```python
from build123d import *

# Parameters (mm, degrees)
SKETCH_2_R           = 2.5
EXTRUDE_4_DEPTH      = 10
SKETCH_3_W           = 45
SKETCH_3_H           = 10
EXTRUDE_5_DEPTH      = 53.5
CUT_EXTRUDE_2_DEPTH  = 62
SKETCH_5_W           = 2
SKETCH_5_H           = 40
EXTRUDE_6_DEPTH      = 4
SKETCH_6_W           = 6
SKETCH_6_H           = 18.13920413
SKETCH_6_H_2         = 19.86079587
EXTRUDE_7_DEPTH      = 2
SKETCH_8_R           = 2
CUT_EXTRUDE_3_DEPTH  = 15
SKETCH_9_W           = 4
SKETCH_9_H           = 2
CUT_EXTRUDE_4_DEPTH  = 8
CUT_EXTRUDE_6_DEPTH  = 70.189906512
CUT_EXTRUDE_7_DEPTH  = 70.189906512
CUT_EXTRUDE_8_DEPTH  = 4
CHAMFER_1_SIZE       = 0.5
CHAMFER_2_SIZE       = 1
FILLET_1_R           = 1
FILLET_2_R           = 1
SKETCH_13_R          = 2.65
CUT_EXTRUDE_9_DEPTH  = 74.226354795
CUT_EXTRUDE_10_DEPTH = 62
SKETCH_15_R          = 2.15
CUT_EXTRUDE_11_DEPTH = 15
SKETCH_16_W          = 9
SKETCH_16_H          = 5
CUT_EXTRUDE_12_DEPTH = 8.5


with BuildPart() as part:
    # Эскиз2 → Бобышка-Вытянуть4 (new body)
    with BuildSketch(Plane.XY):
        with BuildLine():
            Line((-25.592834214, -15.977988248), (-13.092834214, -15.977988248))
            ThreePointArc((-13.092834214, -15.977988248), (-3.092834214, -5.977988248), (6.907165786, -15.977988248))
            Line((6.907165786, -15.977988248), (19.407165786, -15.977988248))
            Line((19.407165786, -15.977988248), (19.407165786, -25.977988248))
            Line((19.407165786, -25.977988248), (-25.592834214, -25.977988248))
            Line((-25.592834214, -25.977988248), (-25.592834214, -15.977988248))
        make_face()
        with Locations((-3.092834214, -15.977988248)):
            Circle(SKETCH_2_R, mode=Mode.SUBTRACT)
    extrude(amount=EXTRUDE_4_DEPTH)

    # Эскиз3 → Бобышка-Вытянуть5 (add)
    with BuildSketch(Plane.XY.offset(10)):
        with Locations((-3.092834214, -20.977988248)):
            Rectangle(SKETCH_3_W, SKETCH_3_H)
    extrude(amount=EXTRUDE_5_DEPTH)

    # Эскиз4 → Вырез-Вытянуть2 (cut)
    with BuildSketch(Plane.XY.offset(63.5)):
        Polygon((-0.783433137, -19.977988248), (1.52596794, -15.977988248), (-0.783433137, -11.977988248), (-5.40223529, -11.977988248), (-7.711636367, -15.977988248), (-5.40223529, -19.977988248), align=None)
    extrude(amount=-CUT_EXTRUDE_2_DEPTH, mode=Mode.SUBTRACT)

    # Эскиз5 → Бобышка-Вытянуть6 (add)
    with BuildSketch(Plane(origin=(0, -15.977988248, 0), x_dir=(1, 0, 0), z_dir=(0, 1, 0))):
        with Locations((-22.092834214, -20)):
            Rectangle(SKETCH_5_W, SKETCH_5_H)
        Polygon((-13.092834214, 0), (-15.092834214, 0), (-15.092834214, -40), (-13.092834214, -40), (-13.092834214, -10), align=None)
    extrude(amount=EXTRUDE_6_DEPTH)

    # Эскиз6 → Бобышка-Вытянуть7 (add)
    with BuildSketch(Plane(origin=(0, -11.977988248, 0), x_dir=(1, 0, 0), z_dir=(0, 1, 0))):
        with Locations((-16.092834214, -9.069602065)):
            Rectangle(SKETCH_6_W, SKETCH_6_H)
        with Locations((-20.092834214, -30.069602065)):
            Rectangle(SKETCH_6_W, SKETCH_6_H_2)
    extrude(amount=EXTRUDE_7_DEPTH)

    # Эскиз8 → Вырез-Вытянуть3 (cut)
    with BuildSketch(Plane(origin=(0, 0, 0), x_dir=(-1, 0, 0), z_dir=(0, 0, -1))):
        with Locations((-12.407165786, -21.977988248)):
            Circle(SKETCH_8_R)
        with Locations((18.592834214, -21.977988248)):
            Circle(SKETCH_8_R)
    extrude(amount=-CUT_EXTRUDE_3_DEPTH, mode=Mode.SUBTRACT)

    # Эскиз9 → Вырез-Вытянуть4 (cut)
    with BuildSketch(Plane.XZ.offset(25.977988248)):
        Polygon((12.407165786, 8), (12.407165786, 10), (12.407165786, 12), (8.407165786, 12), (8.407165786, 8), align=None)
        with Locations((14.407165786, 9)):
            Rectangle(SKETCH_9_W, SKETCH_9_H)
        with Locations((14.407165786, 11)):
            Rectangle(SKETCH_9_W, SKETCH_9_H)
        Polygon((-18.592834214, 12), (-14.592834214, 12), (-14.592834214, 8), (-22.592834214, 8), (-22.592834214, 12), align=None)
    extrude(amount=-CUT_EXTRUDE_4_DEPTH, mode=Mode.SUBTRACT)

    # Эскиз10 → Вырез-Вытянуть6 (cut, through all)
    with BuildSketch(Plane(origin=(0, -15.977988248, 0), x_dir=(1, 0, 0), z_dir=(0, 1, 0))):
        with BuildLine():
            Line((5.466566863, -53.5), (5.466566863, -25))
            ThreePointArc((5.466566863, -25), (10.466566863, -20), (15.466566863, -25))
            Line((15.466566863, -25), (15.466566863, -53.5))
            ThreePointArc((15.466566863, -53.5), (10.466566863, -58.5), (5.466566863, -53.5))
        make_face()
    extrude(amount=-CUT_EXTRUDE_6_DEPTH, mode=Mode.SUBTRACT)

    # Эскиз11 → Вырез-Вытянуть7 (cut, through all)
    with BuildSketch(Plane(origin=(0, -15.977988248, 0), x_dir=(1, 0, 0), z_dir=(0, 1, 0))):
        with BuildLine():
            Line((-21.842834214, -52.5), (-21.842834214, -59))
            ThreePointArc((-21.842834214, -59), (-20.342834214, -60.5), (-18.842834214, -59))
            Line((-18.842834214, -59), (-18.842834214, -52.5))
            ThreePointArc((-18.842834214, -52.5), (-20.342834214, -51), (-21.842834214, -52.5))
        make_face()
        with BuildLine():
            Line((-15.342834214, -52.5), (-15.342834214, -59))
            ThreePointArc((-15.342834214, -59), (-13.842834214, -60.5), (-12.342834214, -59))
            Line((-12.342834214, -59), (-12.342834214, -52.5))
            ThreePointArc((-12.342834214, -52.5), (-13.842834214, -51), (-15.342834214, -52.5))
        make_face()
    extrude(amount=-CUT_EXTRUDE_7_DEPTH, mode=Mode.SUBTRACT)

    # Эскиз12 → Вырез-Вытянуть8 (cut)
    with BuildSketch(Plane.XZ.offset(25.977988248)):
        with BuildLine():
            Line((-23.142834214, 59), (-23.142834214, 52.5))
            ThreePointArc((-23.142834214, 52.5), (-20.342834214, 49.7), (-17.542834214, 52.5))
            Line((-17.542834214, 52.5), (-17.542834214, 59))
            ThreePointArc((-17.542834214, 59), (-20.342834214, 61.8), (-23.142834214, 59))
        make_face()
        with BuildLine():
            Line((-16.642834214, 52.5), (-16.642834214, 59))
            ThreePointArc((-16.642834214, 59), (-13.842834214, 61.8), (-11.042834214, 59))
            Line((-11.042834214, 59), (-11.042834214, 52.5))
            ThreePointArc((-11.042834214, 52.5), (-13.842834214, 49.7), (-16.642834214, 52.5))
        make_face()
    extrude(amount=-CUT_EXTRUDE_8_DEPTH, mode=Mode.SUBTRACT)

    # Фаска1
    # the kernel refuses this chamfer: 0.5 mm, written as the material it takes off along each edge
    with BuildSketch(Plane(origin=(-20.342834214, -25.977988248, 59), x_dir=(1, 0, 0), z_dir=(0, 0, -1))) as chamfer_1_piece_1:
        Polygon((2.8 + CHAMFER_1_SIZE, 0), (2.8, -CHAMFER_1_SIZE), (2.8, 0), align=None)
    revolve(axis=Axis((-20.342834214, -25.977988248, 59), (0, -1, 0)), revolution_arc=180, mode=Mode.SUBTRACT)
    with BuildSketch(Plane(origin=(-23.142834214, -25.977988248, 59), x_dir=(-0.9996219169112968, -0.027495876610589005, 0), z_dir=(0, 0, -1)), Plane(origin=(-17.542834214, -25.977988248, 52.5), x_dir=(0.9996219169112968, -0.027495876610589196, 0), z_dir=(0, 0, 1))) as chamfer_1_piece_2:
        Polygon((CHAMFER_1_SIZE * 0.999621916911, CHAMFER_1_SIZE * 0.0274958766106), (-CHAMFER_1_SIZE * 0.0274958766106, CHAMFER_1_SIZE * 0.999621916911), (0, 0), align=None)
    extrude(amount=6.5, mode=Mode.SUBTRACT)
    with BuildSketch(Plane(origin=(-20.342834214, -25.977988248, 52.5), x_dir=(-1, 0, 0), z_dir=(0, 0, 1))) as chamfer_1_piece_3:
        Polygon((2.8 + CHAMFER_1_SIZE, 0), (2.8, -CHAMFER_1_SIZE), (2.8, 0), align=None)
    revolve(axis=Axis((-20.342834214, -25.977988248, 52.5), (0, -1, 0)), revolution_arc=180, mode=Mode.SUBTRACT)
    with BuildSketch(Plane(origin=(-13.842834214, -25.977988248, 52.5), x_dir=(1, 0, 0), z_dir=(0, 0, 1))) as chamfer_1_piece_4:
        Polygon((2.8 + CHAMFER_1_SIZE, 0), (2.8, CHAMFER_1_SIZE), (2.8, 0), align=None)
    revolve(axis=Axis((-13.842834214, -25.977988248, 52.5), (0, 1, 0)), revolution_arc=180, mode=Mode.SUBTRACT)
    with BuildSketch(Plane(origin=(-11.042834214, -25.977988248, 59), x_dir=(0.9996219169112968, -0.0274958766105891, 0), z_dir=(0, 0, -1)), Plane(origin=(-16.642834214, -25.977988248, 52.5), x_dir=(-0.9996219169112968, -0.027495876610589005, 0), z_dir=(0, 0, 1))) as chamfer_1_piece_5:
        Polygon((CHAMFER_1_SIZE * 0.999621916911, -CHAMFER_1_SIZE * 0.0274958766106), (-CHAMFER_1_SIZE * 0.0274958766106, -CHAMFER_1_SIZE * 0.999621916911), (0, 0), align=None)
    extrude(amount=6.5, mode=Mode.SUBTRACT)
    with BuildSketch(Plane(origin=(-13.842834214, -25.977988248, 59), x_dir=(-1, 0, 0), z_dir=(0, 0, -1))) as chamfer_1_piece_6:
        Polygon((2.8 + CHAMFER_1_SIZE, 0), (2.8, CHAMFER_1_SIZE), (2.8, 0), align=None)
    revolve(axis=Axis((-13.842834214, -25.977988248, 59), (0, 1, 0)), revolution_arc=180, mode=Mode.SUBTRACT)

    # Фаска2
    chamfer_2_edges = [part.edges().sort_by_distance(p)[0] for p in [
        (-25.592834214, -15.977988248, 31.75),
        (19.407165786, -15.977988248, 31.75),
        (19.407165786, -25.977988248, 31.75),
        (-25.592834214, -25.977988248, 31.75),
        (-25.592834214, -20.977988248, 63.5),
        (-3.092834214, -25.977988248, 63.5),
        (10.466566863, -15.977988248, 63.5),
        (-16.65223529, -15.977988248, 63.5),
        (0.371267401, -17.977988248, 63.5),
        (-6.556935829, -17.977988248, 63.5),
        (-3.092834214, -19.977988248, 63.5),
    ]]
    chamfer(chamfer_2_edges, length=CHAMFER_2_SIZE)

    # Скругление1
    fillet_1_edges = [part.edges().sort_by_distance(p)[0] for p in [
        (5.466566863, -15.977988248, 39.25),
        (15.466566863, -15.977988248, 39.25),
        (10.466566863, -15.977988248, 58.5),
        (10.466566863, -15.977988248, 20),
    ]]
    fillet(fillet_1_edges, radius=FILLET_1_R)

    # Скругление2
    fillet_2_edges = [part.edges().sort_by_distance(p)[0] for p in [
        (10.466566863, -25.977988248, 20),
        (10.466566863, -25.977988248, 58.5),
        (5.466566863, -25.977988248, 39.25),
        (15.466566863, -25.977988248, 39.25),
    ]]
    fillet(fillet_2_edges, radius=FILLET_2_R)

    # Эскиз13 → Вырез-Вытянуть9 (cut, through all)
    with BuildSketch(Plane(origin=(0, 0, 0), x_dir=(-1, 0, 0), z_dir=(0, 0, -1))):
        with Locations((3.092834214, -15.977988248)):
            Circle(SKETCH_13_R)
    extrude(amount=-CUT_EXTRUDE_9_DEPTH, mode=Mode.SUBTRACT)

    # Эскиз14 → Вырез-Вытянуть10 (cut)
    with BuildSketch(Plane.XY.offset(63.5)):
        Polygon((1.699173021, -15.977988248), (-0.696830597, -11.827988248), (-5.488837831, -11.827988248), (-7.884841448, -15.977988248), (-5.488837831, -20.127988248), (-0.696830597, -20.127988248), align=None)
    extrude(amount=-CUT_EXTRUDE_10_DEPTH, mode=Mode.SUBTRACT)

    # Эскиз15 → Вырез-Вытянуть11 (cut)
    with BuildSketch(Plane(origin=(0, 0, 0), x_dir=(-1, 0, 0), z_dir=(0, 0, -1))):
        with Locations((18.592834214, -21.977988248)):
            Circle(SKETCH_15_R)
        with Locations((-12.407165786, -21.977988248)):
            Circle(SKETCH_15_R)
    extrude(amount=-CUT_EXTRUDE_11_DEPTH, mode=Mode.SUBTRACT)

    # Эскиз16 → Вырез-Вытянуть12 (cut)
    with BuildSketch(Plane.XZ.offset(25.977988248)):
        with Locations((12.407165786, 10)):
            Rectangle(SKETCH_16_W, SKETCH_16_H)
        with Locations((-18.592834214, 10)):
            Rectangle(SKETCH_16_W, SKETCH_16_H)
    extrude(amount=-CUT_EXTRUDE_12_DEPTH, mode=Mode.SUBTRACT)


solid = part.part
```
Can you work these out from the model? Positions are in its coordinate system, mm. A direction names the side the tool comes from. Coordinates: 2 decimals unless noted, no trailing zeros. Order: outer loops, then holes, each group sorted by start corner. A loop starts at its lowest first (then second) coordinate and runs counter-clockwise, first axis right, second up.
1. Thinking about a two-plate mould opening in Z: for faces 1 (the face through (-6.67, -13.87, 5.81)), 2 (the face through (-13.8, -18.9, 51)), 3 (the face through (-19, -22, 15)), 4 (the face through (-20.3, -23.8, 61.8)), which applies, +Z half, -Z half, draft (parallel to the pull), parting line (faces both ways), or undercut?
2. I'm going to push flat-ended pins straight in: pin 1 (10 mm diameter, centred on y = -11.5, z = 18, fed in from -X); pin 2 (1 mm diameter, centred on x = 11.5, y = -21, fed in from -Z); pin 3 (1 mm diameter, centred on x = 5.5, z = 47, fed in from +Y). Where does each tip first touch, or does it pass through?
3. For faces 5 (the face through (-21.093, -14, 20)), 6 (the face through (-21.5, -12.4, 40)), 7 (the face through (-23.093, -22, 10)), 8 (the face through (-22, -11.978, 10)), which set-ups out of +Z, -Z, +X, -X, +Y, -Y let a thin tool reach every point of the face, with its end or its side?
4. If we section it at B-B (z = 44.5): Please give me the cut outline in (x, y), then the cut area to 3 significant figures.
5. I need wall thicknesses on line 1 (X direction, y = -23.5, z = 28); line 2 (Z direction, x = -17, y = -20); line 3 (X direction, y = -19.5, z = 25.5). Which ranges of each line are inside material? Lowest first, please.
6. If we section it at D-D (x = -7): Please give me the cut outline in (y, z), then the cut area to 3 significant figures.
Entries:
1. face 1: draft
1. face 2: undercut
1. face 3: -Z half
1. face 4: undercut
2. pin 1: stops at x = -25.11
2. pin 2: stops at z = 15
2. pin 3: stops at y = -16.13
3. face 5: +Z, -Z
3. face 6: +Z, +X, -X, +Y
3. face 7: -Y
3. face 8: -Z, -X, +Y
4. outline: (-25.59, -24.98) - (-24.59, -25.98) - (4.47, -25.98) arc R1 ccw to (5.47, -24.98) - (5.47, -16.98) arc R1 ccw to (4.47, -15.98) - (1.7, -15.98) - (-0.7, -20.13) - (-5.49, -20.13) - (-7.88, -15.98) - (-24.59, -15.98) - (-25.59, -16.98) - close; (15.47, -24.98) arc R1 ccw to (16.47, -25.98) - (18.41, -25.98) - (19.41, -24.98) - (19.41, -16.98) - (18.41, -15.98) - (16.47, -15.98) arc R1 ccw to (15.47, -16.98) - close
4. area: 317 mm2
5. line 1: x = -25.59 to 5.47, 15.47 to 19.41
5. line 2: z = 0 to 7.5, 12.5 to 63.5
5. line 3: x = -25.59 to -5.85, -0.33 to 5.47, 15.47 to 19.41
6. outline: (-25.98, 0) - (-6.77, 0) - (-6.77, 10) - (-14.45, 10) - (-14.45, 1.5) - (-17.51, 1.5) - (-17.51, 62.65) - (-19.21, 63.5) - (-24.98, 63.5) - (-25.98, 62.5) - close
6. area: 618 mm2
